```python
from build123d import *

# Parameters (mm, degrees)
BOSS_EXTRUDE1_DEPTH     = 6.35
SKETCH2_R               = 3.3734375
CUT_EXTRUDE1_DEPTH      = 49.087533302
CUT_EXTRUDE3_DEPTH      = 49.087533302
CUT_EXTRUDE3_DEPTH_BACK = 49.087533302


with BuildPart() as part:
    # Sketch1 → Boss-Extrude1 (new, symmetric)
    with BuildSketch(Plane.XY):
        with BuildLine():
            Line((0, -23.8125), (40.3352, -23.8125))
            Line((40.3352, -23.8125), (40.3352, -25.4))
            Line((40.3352, -25.4), (0, -25.4))
            ThreePointArc((0, -25.4), (-17.960512242, 17.960512242), (25.4, 0))
            Line((25.4, 0), (25.4, -18.2499))
            ThreePointArc((25.4, -18.2499), (25.864967985, -19.372432015), (26.9875, -19.8374))
            Line((26.9875, -19.8374), (40.3352, -19.8374))
            Line((40.3352, -19.8374), (40.3352, -21.4249))
            Line((40.3352, -21.4249), (26.9875, -21.4249))
            ThreePointArc((26.9875, -21.4249), (24.74243597, -20.49496403), (23.8125, -18.2499))
            Line((23.8125, -18.2499), (23.8125, 0))
            ThreePointArc((23.8125, 0), (-16.837980227, 16.837980227), (0, -23.8125))
        make_face()
    extrude(amount=BOSS_EXTRUDE1_DEPTH, both=True)

    # Sketch2 → Cut-Extrude1 (cut, through all)
    with BuildSketch(Plane(origin=(0, 0, 0), x_dir=(1, 0, 0), z_dir=(0, 1, 0))):
        with Locations(Location((34.925, 0, 0), (0, 0, 270))):
            Circle(SKETCH2_R)
    extrude(amount=-CUT_EXTRUDE1_DEPTH, mode=Mode.SUBTRACT)

    # Sketch4 → Cut-Extrude3 (cut, two sides: drawn at the far end of the back side and taken through both)
    with BuildSketch(Plane(origin=(0, 0, 0), x_dir=(1, 0, 0), z_dir=(0, 1, 0)).offset(-CUT_EXTRUDE3_DEPTH_BACK)):
        with BuildLine():
            Line((-38.72359939, 123.366595742), (38.4302, 6.35))
            ThreePointArc((38.4302, 6.35), (40.3352, 0), (38.4302, -6.35))
            Line((38.4302, -6.35), (-38.72359939, -123.366595742))
            Line((-38.72359939, -123.366595742), (241.601871727, -123.366595742))
            Line((241.601871727, -123.366595742), (241.601871727, 123.366595742))
            Line((241.601871727, 123.366595742), (-38.72359939, 123.366595742))
        make_face()
    extrude(amount=CUT_EXTRUDE3_DEPTH + CUT_EXTRUDE3_DEPTH_BACK, mode=Mode.SUBTRACT)


solid = part.part
```
Source: CAD feature listing. Evaluate the final solid. Frame: model axes, mm. A direction names the side the tool comes from. Round coordinates to 2 decimals unless told otherwise and drop trailing zeros. Write each loop counter-clockwise with the first axis right and the second up, starting at its lowest first coordinate (ties: lowest second). Pieces come first, ordered by that corner, then holes. Notation, with made-up numbers: M -22,50 L 32,50 A34 cw 32,81 Z; hole C 67,-21.75 d10. An arc over 180 degrees is marked long. Answer as a JSON object with one key per item and string values. Group by question number.
(1) Section query B-B on y = -16. Output: boundary loops of the cut face in (x, z), then the cut area to 3 significant figures.
(2) Section query C-C on x = 12. Output: boundary loops of the cut face in (y, z), then the cut area to 3 significant figures.
(3) Reachability of faces 5 (the flat face through (20, -23.812, 0)), 6 (the flat face through (23.812, -9, 0)), 7 (the flat face through (4, -24, 6.35)), 8 (the flat face through (31, -19.837, 0)) from +Z, -Z, +X, -X, +Y, -Y: full face, straight path, thin tool, end or side. Return the list, or none.
(4) Mould query, pull axis X, two halves, no side actions, for faces 1 (the cylindrical face through (-18.54, 17.36, 0.09)), 2 (the cylindrical face through (24.77, -20.52, 0.09)), 3 (the flat face through (25.4, -9, 0)), 4 (the flat face through (4, -24, -6.35)). Classes: +X half, -X half, draft (parallel to the pull), parting line (faces both ways), or undercut.
(5) Section query A-A on z = 0. State how many separate pieces and enclosed holes the cut face has, then the cut area to 3 significant figures.
(6) First-contact query: pin 1 (1.5 mm diameter, centred on y = 2.5, z = 2.5, fed in from -X); pin 2 (3 mm diameter, centred on x = -11.5, z = 2.5, fed in from -Y); pin 3 (4 mm diameter, centred on x = 19.5, z = -1.5, fed in from +Y); pin 4 (6 mm diameter, centred on x = 34.925, z = 0, fed in from -Y). Flat tips, straight axial feed; report the tip coordinate or a pass-through.
(7) Ray query, line 1 (Y direction, x = 31, z = -0.5); line 2 (X direction, y = 0, z = -2.5); line 3 (Y direction, x = 11, z = 0). Return the intervals inside material, ascending. Write a range as [from, to].
Computed values:
{
 "1": {"outline": "M -19.73,-6.35 L -17.64,-6.35 L -17.64,6.35 L -19.73,6.35 Z; M 23.81,-6.35 L 25.4,-6.35 L 25.4,6.35 L 23.81,6.35 Z", "area": "46.7 mm^2"},
 "2": {"outline": "M -25.4,-6.35 L -23.81,-6.35 L -23.81,6.35 L -25.4,6.35 Z; M 20.57,-6.35 L 22.39,-6.35 L 22.39,6.35 L 20.57,6.35 Z", "area": "43.3 mm^2"},
 "3": {"face 5": "+Z, -Z, +X", "face 6": "+Z, -Z", "face 7": "+Z, +X, -X, +Y, -Y", "face 8": "+Z, -Z, +X, +Y"},
 "4": {"face 1": "parting line", "face 2": "undercut", "face 3": "+X half", "face 4": "draft"},
 "5": {"separate pieces": "3", "enclosed holes": "0", "area": "283 mm^2"},
 "6": {"pin 1": "x = -25.34", "pin 2": "y = -23.35", "pin 3": "y = 18.41", "pin 4": "through"},
 "7": {"line 1": "[-25.4, -23.81], [-21.42, -19.84]", "line 2": "[-25.4, -23.81], [23.81, 25.4]", "line 3": "[-25.4, -23.81], [21.12, 22.89]"}
}
